The listing builds one solid part. Answer for the finished solid, in the listing's coordinates (mm). A direction names the side the tool comes from. Coordinates: 2 decimals unless noted, no trailing zeros. Loops run counter-clockwise (first coordinate to the right, second up) from the corner with the lowest first, then second, coordinate; pieces in that order, holes last. Notation, with made-up numbers: M 38,12 L 71,12 A9 ccw 71,25 Z; hole C -33,20 d7. An arc over 180 degrees is marked long. Answer as a JSON object with one key per item and string values. Group by question number.
1. A cutting plane is placed at D-D on x = -23. Give the vertices of the cut face in (y, z), and give its area (3 significant figures).
2. A cutting plane is placed at B-B on x = 0. Give the vertices of the cut face in (y, z).
3. Given pin 1 (7 mm diameter, centred on x = 19, y = -8.5, fed in from +Z); pin 2 (3 mm diameter, centred on y = 27.5, z = 1, fed in from +X); pin 3 (2 mm diameter, centred on y = 25.5, z = 1.5, fed in from -X), each flat-ended and moving along its own axis, determine where each tip first touches the part or whether it passes through.
4. For faces 1 (the face through (26, -9.145, 1.252)), 2 (the face through (11.1, -41.2, 2.54)), 3 (the face through (-8.486, -6.507, 5.009)), 4 (the face through (11, -11, 0)), 5 (the face through (0, 42, 12.7)), determine the directions among +Z, -Z, +X, -X, +Y, -Y from which every point of the face is accessible in a straight line to the end or side of a thin tool.
5. Straight lines are drawn through the part: L1, parallel to Y at x = 0, z = 6; L2, parallel to Y at x = -8.5, z = 2; L3, parallel to X at y = 17.5, z = 1.5. For each, find the intervals that lie inside material, in ascending order.
6. A cutting plane is placed at C-C on y = -6. Give the vertices of the cut face in (x, z).
7. Determine the mould class of faces 6 (the face through (-11.012, -49.592, 1.252)), 7 (the face through (0, 0, 12.7)), 8 (the face through (36.46, 21.68, 1.25)) for opening direction X: released by +X, released by -X, zero draft, split by the parting line, or undercut.
8. A cutting plane is placed at A-A on z = 9. Give the vertices of the cut face in (x, y).
from build123d import *

# Parameters (mm, degrees)
F1_DEPTH = 2.54
F0_R     = 50.8
F2_DEPTH = 12.7
F3_R     = 10.6934
F4_DEPTH = 10.16


with BuildPart() as f1:
    # F0 (on Top) → F1 (new body)
    with BuildSketch(Plane.XY):
        with BuildLine():
            ThreePointArc((-7.5403124952, -10.2192801838), (-10.9985226281, -6.35), (-12.6203124952, -1.4204620814))
            Line((-12.6203124952, -1.4204620814), (-39.0106764813, -16.6569458328))
            ThreePointArc((-39.0106764812, -16.6569458328), (-34.0593747907, -16.8799953872), (-31.6459004079, -21.209))
            ThreePointArc((-31.6459004079, -21.209), (-32.2533470771, -23.6201825743), (-33.9306764813, -25.4557639352))
            Line((-33.9306764813, -25.4557639352), (-7.5403124952, -10.2192801838))
        make_face()
    extrude(amount=F1_DEPTH)



with BuildPart() as f1b:
    # F0 (on Top) → F1, piece 2 (new body)
    with BuildSketch(Plane.XY):
        Circle(F0_R)
        with BuildLine():
            ThreePointArc((-39.0106764812, -16.6569458328), (-36.7350655777, 21.209), (-5.08, 42.112709768))
            ThreePointArc((-5.08, 42.112709768), (-0.1527138878, 47.5048733613), (5.0891651698, 42.418))
            ThreePointArc((5.0891651698, 42.418), (5.0868733613, 42.2652861122), (5.08, 42.112709768))
            ThreePointArc((5.08, 42.112709768), (36.7350655777, 21.209), (39.0106764812, -16.6569458328))
            ThreePointArc((39.0106764813, -16.6569458328), (41.0640701906, -18.533309213), (41.8242307476, -21.209))
            ThreePointArc((41.8242307476, -21.209), (39.146248152, -25.6907185007), (33.9306764812, -25.4557639352))
            ThreePointArc((33.9306764812, -25.4557639352), (0, -42.418), (-33.9306764812, -25.4557639352))
            ThreePointArc((-33.9306764813, -25.4557639352), (-41.1424118989, -23.7535825849), (-39.0106764812, -16.6569458328))
        make_face(mode=Mode.SUBTRACT)
    extrude(amount=F1_DEPTH)


with BuildPart() as f1c:
    # F0 (on Top) → F1, piece 3 (new body)
    with BuildSketch(Plane.XY):
        with BuildLine():
            ThreePointArc((33.9306764812, -25.4557639352), (32.3277192566, -18.6644174151), (39.0106764813, -16.6569458328))
            Line((39.0106764813, -16.6569458328), (12.6203124952, -1.4204620814))
            ThreePointArc((12.6203124952, -1.4204620814), (10.9985226281, -6.35), (7.5403124952, -10.2192801838))
            Line((7.5403124952, -10.2192801838), (33.9306764812, -25.4557639352))
        make_face()
    extrude(amount=F1_DEPTH)


with BuildPart() as f1d:
    # F0 (on Top) → F1, piece 4 (new body)
    with BuildSketch(Plane.XY):
        with BuildLine():
            Line((-5.08, 42.112709768), (-5.08, 11.6397422652))
            ThreePointArc((-5.08, 11.6397422652), (0, 12.7), (5.08, 11.6397422652))
            Line((5.08, 11.6397422652), (5.08, 42.112709768))
            ThreePointArc((5.08, 42.112709768), (0, 37.3288348302), (-5.08, 42.112709768))
        make_face()
    extrude(amount=F1_DEPTH)


with BuildPart() as f1_1:
    add(f1.part)

    add(f1b.part)  # F2 merges F1b

    add(f1c.part)  # F2 merges F1c

    add(f1d.part)  # F2 merges F1d
    # F0 (on Top) → F2 (join)
    with BuildSketch(Plane.XY):
        with BuildLine():
            ThreePointArc((5.08, 11.6397422652), (0, 12.7), (-5.08, 11.6397422652))
            ThreePointArc((-5.08, 11.6397422652), (-10.9985226281, 6.35), (-12.6203124952, -1.4204620814))
            ThreePointArc((-12.6203124952, -1.4204620814), (-10.9985226281, -6.35), (-7.5403124952, -10.2192801838))
            ThreePointArc((-7.5403124952, -10.2192801838), (0, -12.7), (7.5403124952, -10.2192801838))
            ThreePointArc((7.5403124952, -10.2192801838), (10.9985226281, -6.35), (12.6203124952, -1.4204620814))
            ThreePointArc((12.6203124952, -1.4204620814), (12.680062474, -0.7113477741), (12.7, 0))
            ThreePointArc((12.7, 0), (10.625582337, 6.9560764803), (5.08, 11.6397422652))
        make_face()
        with BuildLine():
            ThreePointArc((-31.6459004079, -21.209), (-34.0593747907, -16.8799953872), (-39.0106764812, -16.6569458328))
            ThreePointArc((-39.0106764812, -16.6569458328), (-41.1424118989, -23.7535825849), (-33.9306764813, -25.4557639352))
            ThreePointArc((-33.9306764813, -25.4557639352), (-32.2533470771, -23.6201825743), (-31.6459004079, -21.209))
        make_face()
        with BuildLine():
            ThreePointArc((41.8242307476, -21.209), (41.0640701906, -18.533309213), (39.0106764813, -16.6569458328))
            ThreePointArc((39.0106764813, -16.6569458328), (32.3277192566, -18.6644174151), (33.9306764812, -25.4557639352))
            ThreePointArc((33.9306764812, -25.4557639352), (39.146248152, -25.6907185007), (41.8242307476, -21.209))
        make_face()
        with BuildLine():
            ThreePointArc((5.0891651698, 42.418), (-0.1527138878, 47.5048733613), (-5.08, 42.112709768))
            ThreePointArc((-5.08, 42.112709768), (0, 37.3288348302), (5.08, 42.112709768))
            ThreePointArc((5.08, 42.112709768), (5.0868733613, 42.2652861122), (5.0891651698, 42.418))
        make_face()
    extrude(amount=F2_DEPTH)

    # F3 (on face) → F4 (cut)
    with BuildSketch(Plane.XY):
        Circle(F3_R)
    extrude(amount=F4_DEPTH, mode=Mode.SUBTRACT)


solid = f1_1.part
From the geometry:
{
 "1": {"outline": "M -45.3,0 L -35.64,0 L -35.64,2.54 L -45.3,2.54 Z; M -19.14,0 L -7.41,0 L -7.41,2.54 L -19.14,2.54 Z; M 35.64,0 L 45.3,0 L 45.3,2.54 L 35.64,2.54 Z", "area": "78.8 mm²"},
 "2": {"outline": "M -50.8,0 L -42.42,0 L -42.42,2.54 L -50.8,2.54 Z; M -12.7,0 L -10.69,0 L -10.69,10.16 L 10.69,10.16 L 10.69,0 L 50.8,0 L 50.8,2.54 L 47.51,2.54 L 47.51,12.7 L 37.33,12.7 L 37.33,2.54 L 12.7,2.54 L 12.7,12.7 L -12.7,12.7 Z"},
 "3": {"pin 1": "stops at z = 2.54", "pin 2": "stops at x = 43.64", "pin 3": "stops at x = -44.5"},
 "4": {"face 1": "+Z, -Z", "face 2": "+Z", "face 3": "-Z", "face 4": "-Z, +X, -X, +Y, -Y", "face 5": "+Z, +X, -X, +Y, -Y"},
 "5": {"L1": "y = -12.7 to -10.69, 10.69 to 12.7, 37.33 to 47.51", "L2": "y = -50.08 to -41.56, -10.77 to -6.49, 6.49 to 9.44, 41.56 to 50.08", "L3": "x = -47.69 to -38.64, -5.08 to 5.08, 38.64 to 47.69"},
 "6": {"outline": "M -50.44,0 L -41.99,0 L -41.99,2.54 L -50.44,2.54 Z; M -20.55,0 L -8.85,0 L -8.85,10.16 L 8.85,10.16 L 8.85,0 L 20.55,0 L 20.55,2.54 L 11.19,2.54 L 11.19,12.7 L -11.19,12.7 L -11.19,2.54 L -20.55,2.54 Z; M 41.99,0 L 50.44,0 L 50.44,2.54 L 41.99,2.54 Z"},
 "7": {"face 6": "split by the parting line", "face 7": "zero draft", "face 8": "undercut"},
 "8": {"outline": "C -36.74,-21.21 d10.18; C 0,0 d25.4; C 0,42.42 d10.18; C 36.74,-21.21 d10.18; hole C 0,0 d21.39"}
}
